Drawing for the job (mm, zero at the part's lowest x, y, z). A direction names the side the tool comes from. Coordinates: 2 decimals unless noted, no trailing zeros. Order: outer loops, then holes, each group sorted by start corner. A loop starts at its lowest first (then second) coordinate and runs counter-clockwise, first axis right, second up.
1) Wall check: L1, parallel to X at y = 66, z = 24; L2, parallel to Y at x = 66.04, z = 46; L3, parallel to X at y = 56, z = 27.5. Give the ranges that are in metal, low to high.
2) Cut at D-D (z = 18.5). List the corners of the cut face in (x, y).
3) Cut at C-C (y = 16). List the corners of the cut face in (x, z).
4) Tool access for the marked faces 1 and 2: list every direction of +Z, -Z, +X, -X, +Y, -Y with a clear straight run to the whole face (end or side of a thin tool).
5) Cut at B-B (x = 35.56). List the corners of the cut face in (y, z).
6) Pin check, flat tips, straight feed: pin 1 Ø1.5 at (x, y) = (17, 46.5) entering from +Z; pin 2 Ø5 at (x, y) = (23.5, 94.5) entering from -Z; pin 3 Ø8 at (x, z) = (87.5, 7) entering from -Y. Stop position of each tip, or through.
7) Mould opens along Y. For the marked faces 3, 4 and 5 say: +Y half, -Y half, draft (parallel to the pull), parting line (faces both ways), or undercut.
8) Cut at A-A (y = 66.04). List the corners of the cut face in (x, z), and give its area (3 significant figures).
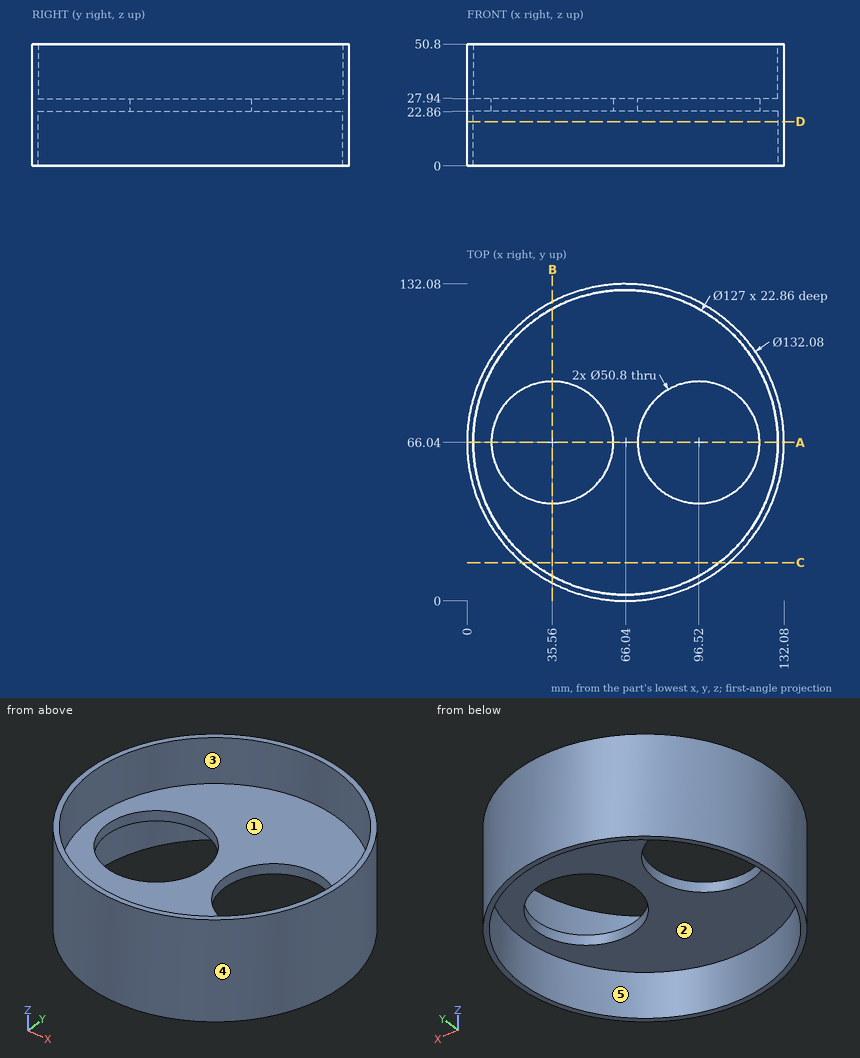
Geometry check:
1. L1: x = 0 to 10.16, 60.96 to 71.12, 121.92 to 132.08
1. L2: y = 0 to 2.54, 129.54 to 132.08
1. L3: x = 0.77 to 12.23, 58.89 to 73.19, 119.85 to 131.31
2. outline: circle Ø132.08 at (66.04, 66.04); hole circle Ø127 at (66.04, 66.04)
3. outline: (22.94, 0) - (26.95, 0) - (26.95, 22.86) - (105.13, 22.86) - (105.13, 0) - (109.14, 0) - (109.14, 50.8) - (105.13, 50.8) - (105.13, 27.94) - (26.95, 27.94) - (26.95, 50.8) - (22.94, 50.8) - close
4. face 1: +Z
4. face 2: -Z
5. outline: (7.45, 0) - (10.33, 0) - (10.33, 22.86) - (40.64, 22.86) - (40.64, 27.94) - (10.33, 27.94) - (10.33, 50.8) - (7.45, 50.8) - close; (91.44, 22.86) - (121.75, 22.86) - (121.75, 0) - (124.63, 0) - (124.63, 50.8) - (121.75, 50.8) - (121.75, 27.94) - (91.44, 27.94) - close
6. pin 1: stops at z = 27.94
6. pin 2: stops at z = 22.86
6. pin 3: stops at y = 2.35
7. face 3: undercut
7. face 4: parting line
7. face 5: undercut
8. outline: (0, 0) - (2.54, 0) - (2.54, 22.86) - (10.16, 22.86) - (10.16, 27.94) - (2.54, 27.94) - (2.54, 50.8) - (0, 50.8) - close; (60.96, 22.86) - (71.12, 22.86) - (71.12, 27.94) - (60.96, 27.94) - close; (121.92, 22.86) - (129.54, 22.86) - (129.54, 0) - (132.08, 0) - (132.08, 50.8) - (129.54, 50.8) - (129.54, 27.94) - (121.92, 27.94) - close
8. area: 387 mm2
